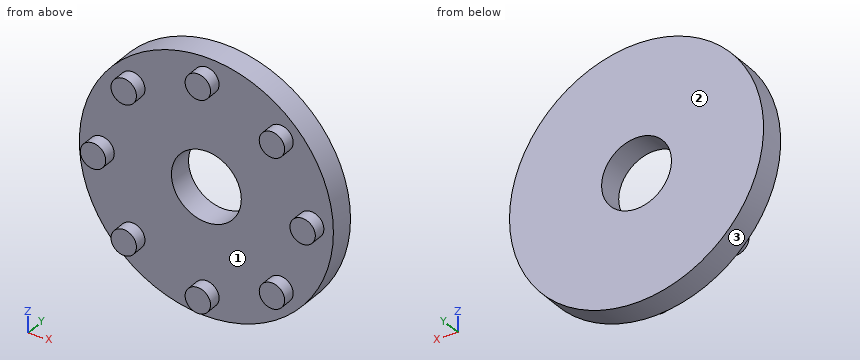
```python
from build123d import *

# Parameters (mm, degrees)
F0_R     = 4
F0_R_2   = 1.1
F1_DEPTH = 0.8
F2_R     = 0.4
F3_DEPTH = 0.4
F4_COUNT = 8


with BuildPart() as f1:
    # F0 (on Front) → F1 (new body)
    with BuildSketch(Plane.XZ):
        Circle(F0_R)
        Circle(F0_R_2, mode=Mode.SUBTRACT)
    extrude(amount=F1_DEPTH)

    # F2 (on face) → F3 (join)
    with BuildSketch(Plane.XZ.offset(0.8)):
        with Locations((0, 3.3)):
            Circle(F2_R)
    extrude(amount=F3_DEPTH)

    # F4: F1 ×8 about axis
    f4_axis = Axis((0, -0.8, 0), (0, -1, 0))


with BuildPart() as f1_1:
    add(f1.part)
    for i in range(1, F4_COUNT):
        add(f1.part.rotate(f4_axis, i * 360 / F4_COUNT))


solid = f1_1.part
```
CAD build for the part. Positions are in the model's coordinates, mm. Face numbers are marked on the shaded views. Round coordinates to 2 decimals unless told otherwise and drop trailing zeros. Write each loop counter-clockwise with the first axis right and the second up, starting at its lowest first coordinate (ties: lowest second). Pieces come first, ordered by that corner, then holes. Notation, with made-up numbers: (-28, -16) - (23, -16) arc R11 ccw to (23, 2) - close; hole circle Ø7 at (70, -26). An arc over 180 degrees is marked (long way). Return JSON: item names as keys, results as strings. Group by question number.
Item 1: Band-saw the part on D-D on y = -0.4. List the corners of the cut face in (x, z).
Item 2: Probe probe 1 along Z at (x, y) = (0, -0.35); probe 2 along X at (y, z) = (-0.7, 3.5). List the from-to ranges inside material, lowest first.
Item 3: Band-saw the part on A-A on z = 0. List the corners of the cut face in (x, y).
Item 4: Mould opens along Z. For the marked faces 1, 2 and 3 say: +Z half, -Z half, draft (parallel to the pull), parting line (faces both ways), or undercut.
Item 5: Band-saw the part on B-B on x = 0. List the corners of the cut face in (y, z).
Item 6: Band-saw the part on C-C on x = -1. List the corners of the cut face in (y, z).
Resolved:
{
 "1": {"outline": "circle Ø8 at (0, 0); hole circle Ø2.2 at (0, 0)"},
 "2": {"probe 1": "z = -4 to -1.1, 1.1 to 4", "probe 2": "x = -1.94 to 1.94"},
 "3": {"outline": "(-4, -0.8) - (-3.7, -0.8) - (-3.7, -1.2) - (-2.9, -1.2) - (-2.9, -0.8) - (-1.1, -0.8) - (-1.1, 0) - (-4, 0) - close; (1.1, -0.8) - (2.9, -0.8) - (2.9, -1.2) - (3.7, -1.2) - (3.7, -0.8) - (4, -0.8) - (4, 0) - (1.1, 0) - close"},
 "4": {"face 1": "undercut", "face 2": "draft", "face 3": "parting line"},
 "5": {"outline": "(-1.2, -3.7) - (-0.8, -3.7) - (-0.8, -4) - (0, -4) - (0, -1.1) - (-0.8, -1.1) - (-0.8, -2.9) - (-1.2, -2.9) - close; (-1.2, 2.9) - (-0.8, 2.9) - (-0.8, 1.1) - (0, 1.1) - (0, 4) - (-0.8, 4) - (-0.8, 3.7) - (-1.2, 3.7) - close"},
 "6": {"outline": "(-0.8, -3.87) - (0, -3.87) - (0, -0.46) - (-0.8, -0.46) - close; (-0.8, 0.46) - (0, 0.46) - (0, 3.87) - (-0.8, 3.87) - close"}
}
